Study the drawing (mm; zero at the part's minimum x, y, z) and answer. A direction names the side the tool comes from. Give positions to 0.01 mm unless a question says otherwise; leave off trailing zeros. One line per question, with ' | ' between items. Start each with the question number.
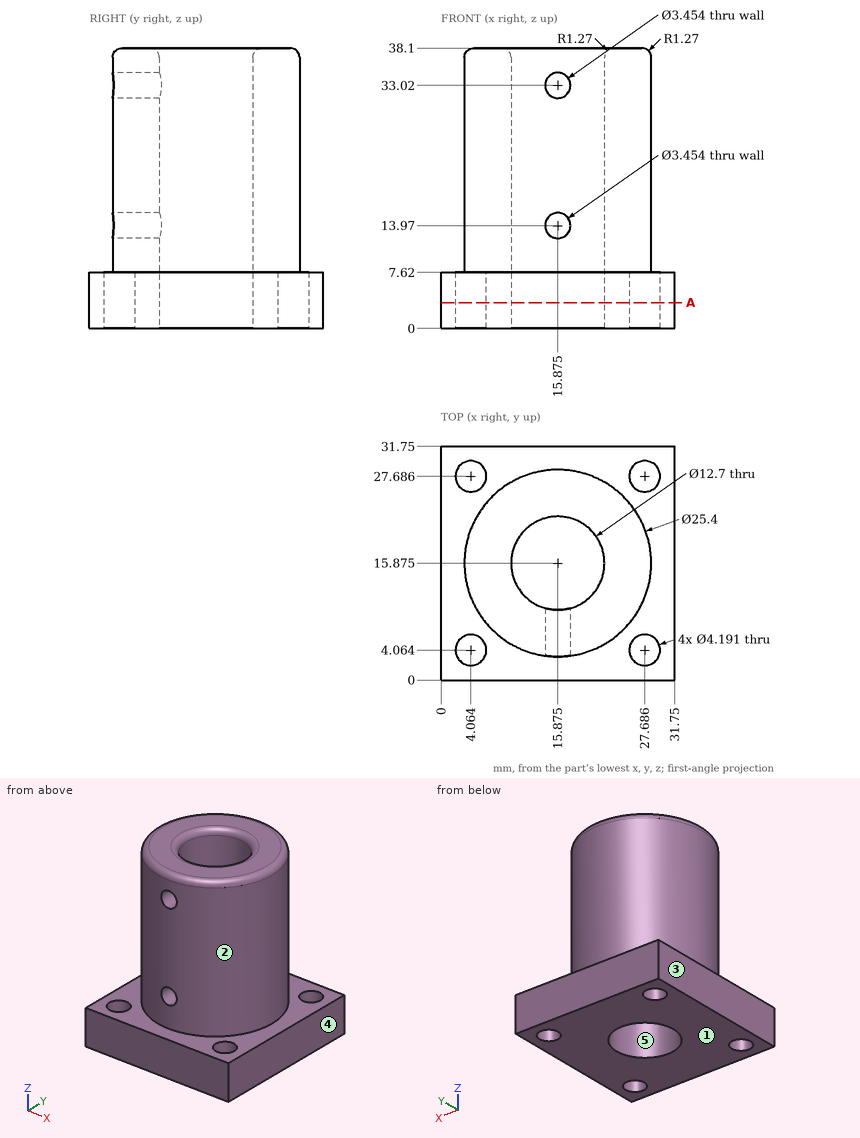
1. Each of these flat-tipped pins is pushed along its axis until it touches: pin 1 Ø1.5 at (x, y) = (25.5, 8) entering from +Z; pin 2 Ø8 at (y, z) = (11.5, 29) entering from -X; pin 3 Ø5 at (x, z) = (17.5, 26) entering from -Y (3 decimals); pin 4 Ø8 at (x, z) = (25.5, 7.5) entering from -Y. Where does it stop, or does it pass through?
2. For the marked faces 1 and 2, determine the directions among +Z, -Z, +X, -X, +Y, -Y from which every point of the face is accessible in a straight line to the end or side of a thin tool.
3. Straight lines are drawn through the part: L1, parallel to X at y = 4, z = 5; L2, parallel to Z at x = 8, y = 29.5; L3, parallel to Y at x = 16, z = 4. For each, find the intervals that lie inside material, in ascending order.
4. Determine the mould class of the marked faces 3, 4 and 5 for opening direction X: released by +X, released by -X, zero draft, split by the parting line, or undercut.
5. The part is cut by section A-A (z = 3.5). Count the separate pieces of the cut face and the enclosed holes in it, plus the area to 3 significant figures.
Check sheet entries:
1) pin 1: stops at z = 38.07 | pin 2: stops at x = 3.18 | pin 3: stops at y = 3.175 | pin 4: stops at y = 0
2) face 1: -Z, +X, -X, +Y, -Y | face 2: +Z
3) L1: x = 0 to 1.97, 6.16 to 25.59, 29.78 to 31.75 | L2: z = 0 to 7.62 | L3: y = 0 to 9.53, 22.22 to 31.75
4) face 3: released by -X | face 4: released by +X | face 5: undercut
5) separate pieces: 1 | enclosed holes: 5 | area: 826 mm^2
